from build123d import *

# Parameters (mm, degrees)
BOSS_EXTRUDE1_DEPTH                     = 450
CHAMFER1_SIZE                           = 0.3
CBORE_FOR_M5_HEX_HEAD_BOLT1_D           = 3.5
CBORE_FOR_M5_HEX_HEAD_BOLT1_CBORE_D     = 6
CBORE_FOR_M5_HEX_HEAD_BOLT1_CBORE_DEPTH = 4.5
LPATTERN1_COUNT                         = 18
LPATTERN1_PITCH                         = 25


with BuildPart() as part:
    # Sketch1 → Boss-Extrude1 (new body)
    with BuildSketch(Plane.XY):
        with BuildLine():
            Line((0, 8), (12, 8))
            Line((12, 8), (12, 6.75))
            Line((12, 6.75), (12, 6.559016994))
            ThreePointArc((12, 6.559016994), (11.706107374, 6.475528258), (11.5, 6.25))
            Line((11.5, 6.25), (11, 6.25))
            Line((11, 6.25), (11, 5.75))
            Line((11, 5.75), (11.5, 5.75))
            ThreePointArc((11.5, 5.75), (11.706107374, 5.524471742), (12, 5.440983006))
            Line((12, 5.440983006), (12, 5.25))
            Line((12, 5.25), (12, 0))
            Line((12, 0), (0, 0))
            Line((0, 0), (0, 5.25))
            Line((0, 5.25), (0, 5.440983006))
            ThreePointArc((0, 5.440983006), (0.293892626, 5.524471742), (0.5, 5.75))
            Line((0.5, 5.75), (1, 5.75))
            Line((1, 5.75), (1, 6.25))
            Line((1, 6.25), (0.5, 6.25))
            ThreePointArc((0.5, 6.25), (0.293892626, 6.475528258), (0, 6.559016994))
            Line((0, 6.559016994), (0, 6.75))
            Line((0, 6.75), (0, 8))
        make_face()
    extrude(amount=BOSS_EXTRUDE1_DEPTH)

    # Chamfer1
    chamfer1_edges = [part.edges().sort_by_distance(p)[0] for p in [
        (12, 2.720491503, 450),
        (11.706107374, 5.524471742, 450),
        (0, 2.720491503, 0),
        (0.293892626, 5.524471742, 0),
        (0.75, 5.75, 0),
        (1, 6, 0),
        (0.75, 6.25, 0),
        (11.25, 5.75, 450),
        (0.293892626, 6.475528258, 0),
        (0, 7.279508497, 0),
        (6, 8, 0),
        (12, 7.279508497, 0),
        (11.706107374, 6.475528258, 0),
        (11, 6, 450),
        (11.25, 6.25, 0),
        (11, 6, 0),
        (11.25, 5.75, 0),
        (11.706107374, 5.524471742, 0),
        (12, 2.720491503, 0),
        (6, 0, 0),
        (11.25, 6.25, 450),
        (11.706107374, 6.475528258, 450),
        (12, 7.279508497, 450),
        (0, 8, 225),
        (12, 8, 225),
        (12, 0, 225),
        (0, 0, 225),
        (6, 8, 450),
        (0, 2.720491503, 450),
        (0, 7.279508497, 450),
        (0.293892626, 6.475528258, 450),
        (0.75, 6.25, 450),
        (1, 6, 450),
        (0.75, 5.75, 450),
        (0.293892626, 5.524471742, 450),
        (6, 0, 450),
    ]]
    chamfer(chamfer1_edges, length=CHAMFER1_SIZE)

    # CBORE for M5 Hex Head Bolt1 (through all)
    with Locations(Plane(origin=(6, 8, 12.5), x_dir=(0, 0, 1), z_dir=(0, 1, 0))):
        with Locations((0, 0)):
            cbore_for_m5_hex_head_bolt1 = CounterBoreHole(CBORE_FOR_M5_HEX_HEAD_BOLT1_D / 2, CBORE_FOR_M5_HEX_HEAD_BOLT1_CBORE_D / 2, CBORE_FOR_M5_HEX_HEAD_BOLT1_CBORE_DEPTH)

    # LPattern1: CBORE for M5 Hex Head Bolt1 ×18
    with Locations(*[(0, 0, i * LPATTERN1_PITCH) for i in range(1, LPATTERN1_COUNT)]):
        add(cbore_for_m5_hex_head_bolt1, mode=Mode.SUBTRACT)


solid = part.part
Model file for the job. Use its own axes, mm. Give positions to 0.01 mm unless a question says otherwise; leave off trailing zeros. Loops run counter-clockwise (first coordinate to the right, second up) from the corner with the lowest first, then second, coordinate; pieces in that order, holes last.
1) Wall check: line 1 (X direction, y = 2.25, z = 287.5); line 2 (X direction, y = 6.9, z = 162.5); line 3 (X direction, y = 5.5, z = 366.5). Give the ranges that are in metal, low to high.
2) Saw through at A-A (y = 1.75). Count the separate pieces of the cut face and the enclosed holes in it, plus the area to 3 significant figures.
3) Flat gauge pin, fed straight in: pin 1 Ø5.5 at (x, z) = (6, 62.5) entering from +Y. Where does the tip first touch, or does it go through?
4) Saw through at B-B (z = 397). Write the cut outline in (x, y).
Answer block:
1. line 1: x = 0 to 4.25, 7.75 to 12
1. line 2: x = 0 to 3, 9 to 12
1. line 3: x = 0.25 to 11.75
2. separate pieces: 1
2. enclosed holes: 18
2. area: 5,230 mm2
3. pin 1: stops at y = 3.5
4. outline: (0, 0.3) - (0.3, 0) - (11.7, 0) - (12, 0.3) - (12, 5.44) arc R0.56 cw to (11.5, 5.75) - (11, 5.75) - (11, 6.25) - (11.5, 6.25) arc R0.56 cw to (12, 6.56) - (12, 7.7) - (11.7, 8) - (0.3, 8) - (0, 7.7) - (0, 6.56) arc R0.56 cw to (0.5, 6.25) - (1, 6.25) - (1, 5.75) - (0.5, 5.75) arc R0.56 cw to (0, 5.44) - close
